The model under review builds one solid part; all positions refer to its coordinate system, in mm. Give positions to 0.01 mm unless a question says otherwise; leave off trailing zeros. Order: outer loops, then holes, each group sorted by start corner. A loop starts at its lowest first (then second) coordinate and runs counter-clockwise, first axis right, second up. Notation, with made-up numbers: (58.25, 78) - (114.25, 78) arc R21 ccw to (114.25, 116) - close; hole circle Ø6 at (15.25, 48). An arc over 180 degrees is marked (long way). Put each result on its own line as item: value.
```python
from build123d import *

# Parameters (mm, degrees)
SKETCH_1_R             = 110
SKETCH_1_R_2           = 68.5
SKETCH_1_R_3           = 8.5
SM_BASE_FLANGE_1_DEPTH = 6


# Sheet-metal steps are written as plain solids
with BuildPart() as part:
    # Sketch 1 → Базовая кромка1 (new body)
    with BuildSketch(Plane.XY):
        Circle(SKETCH_1_R)
        Circle(SKETCH_1_R_2, mode=Mode.SUBTRACT)
        with Locations((77.076260937, 44.5)):
            Circle(SKETCH_1_R_3, mode=Mode.SUBTRACT)
        with Locations((0, -89)):
            Circle(SKETCH_1_R_3, mode=Mode.SUBTRACT)
        with Locations((-77.076260937, 44.5)):
            Circle(SKETCH_1_R_3, mode=Mode.SUBTRACT)
    extrude(amount=-SM_BASE_FLANGE_1_DEPTH)


solid = part.part
```
(1) Take a section at D-D, the plane x = 72. Write out the cut boundary in (y, z), then the cut area to 3 significant figures.
The answers:
outline: (-83.16, -6) - (37.68, -6) - (37.68, 0) - (-83.16, 0) - close; (51.32, -6) - (83.16, -6) - (83.16, 0) - (51.32, 0) - close
area: 916 mm^2
(2) Take a section at B-B, the plane x = 0. Write out the cut boundary in (y, z).
The answers:
outline: (-110, -6) - (-97.5, -6) - (-97.5, 0) - (-110, 0) - close; (-80.5, -6) - (-68.5, -6) - (-68.5, 0) - (-80.5, 0) - close; (68.5, -6) - (110, -6) - (110, 0) - (68.5, 0) - close
(3) Take a section at C-C, the plane z = -3. Write out the cut boundary in (x, y).
The answers:
outline: circle Ø220 at (0, 0); hole circle Ø17 at (-77.08, 44.5); hole circle Ø137 at (0, 0); hole circle Ø17 at (0, -89); hole circle Ø17 at (77.08, 44.5)
(4) Clearance check with a flat-ended pin moving along its axis: pin 1 Ø13.5 at (x, y) = (0, -89) entering from -Z. State where the tip first meets the part, or that it passes through.
The answers:
pin 1: through
(5) The part is to be moulded in two halves that separate along X. For faces 1 (the cylindrical face through (-23.846, -107.384, -2.958)), 2 (the flat face through (-50.4, -47.3, 0)), 3 (the cylindrical face through (65.337, 20.576, -2.958)), say which applies: pulls with the +X half, pulls with the -X half, needs draft (parallel to the pull), parting line crosses it, or undercut.
The answers:
face 1: parting line crosses it
face 2: needs draft
face 3: undercut
(6) Wall thickness on L1, parallel to Y at x = 0, z = -1.5; L2, parallel to Y at x = -6.5, z = -1.4; L3, parallel to X at y = 39, z = -3.75: over which ranges is each line inside the solid? List them lowest first.
The answers:
L1: -110 to -97.5, -80.5 to -68.5, 68.5 to 110
L2: -109.81 to -94.48, -83.52 to -68.19, 68.19 to 109.81
L3: -102.85 to -83.56, -70.6 to -56.31, 56.31 to 70.6, 83.56 to 102.85
(7) Take a section at A-A, the plane y = 0. Write out the cut boundary in (x, z).
The answers:
outline: (-110, -6) - (-68.5, -6) - (-68.5, 0) - (-110, 0) - close; (68.5, -6) - (110, -6) - (110, 0) - (68.5, 0) - close
